CAD build for the part. Positions are in the model's coordinates, mm. A direction names the side the tool comes from. Coordinates: 2 decimals unless noted, no trailing zeros. Loops run counter-clockwise (first coordinate to the right, second up) from the corner with the lowest first, then second, coordinate; pieces in that order, holes last. Notation, with made-up numbers: (65, 70.5) -> (102, 70.5) arc R14 cw to (102, 86.5) -> close; hole circle Ø4 at (-5.5, 79). An arc over 180 degrees is marked (long way). Write each question's results on one line, items separated by ' | '.
from build123d import *

# Parameters (mm, degrees)
SKETCH_1_R      = 1.4
EXTRUDE_1_DEPTH = 33


with BuildPart() as part:
    # 草图1 → 凸台-拉伸1 (new body)
    with BuildSketch(Plane(origin=(0, 0, 0), x_dir=(1, 0, 0), z_dir=(0, 1, 0))):
        with BuildLine():
            Line((63.539198291, -45.541591726), (63.539198291, -25.541591726))
            Line((63.539198291, -25.541591726), (83.539198291, -25.541591726))
            ThreePointArc((83.539198291, -25.541591726), (88.539198291, -20.541591726), (83.539198291, -15.541591726))
            Line((83.539198291, -15.541591726), (49.205502665, -15.541591726))
            ThreePointArc((49.205502665, -15.541591726), (45.669968759, -17.006057821), (44.205502665, -20.541591726))
            Line((44.205502665, -20.541591726), (44.205502665, -50.541591726))
            ThreePointArc((44.205502665, -50.541591726), (45.669968759, -54.077125632), (49.205502665, -55.541591726))
            Line((49.205502665, -55.541591726), (83.539198291, -55.541591726))
            ThreePointArc((83.539198291, -55.541591726), (88.539198291, -50.541591726), (83.539198291, -45.541591726))
            Line((83.539198291, -45.541591726), (63.539198291, -45.541591726))
        make_face()
        with Locations(Location((83.539198291, -20.541591726, 0), (0, 0, 270))):
            Circle(SKETCH_1_R, mode=Mode.SUBTRACT)
        with Locations(Location((83.539198291, -50.541591726, 0), (0, 0, 90))):
            Circle(SKETCH_1_R, mode=Mode.SUBTRACT)
        with Locations(Location((51.406078432, -20.541591726, 0), (0, 0, 270))):
            Circle(SKETCH_1_R, mode=Mode.SUBTRACT)
        with Locations(Location((51.406078432, -35.541591726, 0), (0, 0, 270))):
            Circle(SKETCH_1_R, mode=Mode.SUBTRACT)
        with Locations(Location((51.406078432, -50.541591726, 0), (0, 0, 90))):
            Circle(SKETCH_1_R, mode=Mode.SUBTRACT)
    extrude(amount=EXTRUDE_1_DEPTH)


solid = part.part
1) Slice it at A-A (x = 67). Write the cut outline in (y, z).
Outcome:
outline: (0, 15.54) -> (33, 15.54) -> (33, 25.54) -> (0, 25.54) -> close; (0, 45.54) -> (33, 45.54) -> (33, 55.54) -> (0, 55.54) -> close
2) Pin check, flat tips, straight feed: pin 1 (6 mm diameter, centred on y = 24.5, z = 39.5, fed in from +X); pin 2 (1.7 mm diameter, centred on x = 83.54, z = 20.54, fed in from -Y); pin 3 (12 mm diameter, centred on y = 26.5, z = 28.5, fed in from +X). Stop position of each tip, or through.
Outcome:
pin 1: stops at x = 63.54 | pin 2: passes through | pin 3: stops at x = 88.14
3) Drill centre lines: L1, parallel to Z at x = 74, y = 21.5; L2, parallel to Z at x = 83.5, y = 22; L3, parallel to X at y = 4, z = 19.5. Where is each one in solid material? Low to high. Write a range as from..to.
Outcome:
L1: z = 15.54..25.54, 45.54..55.54 | L2: z = 15.54..19.14, 21.94..25.54, 45.54..49.14, 51.94..55.54 | L3: x = 44.32..50.47, 52.34..82.6, 84.47..88.43
4) Slice it at C-C (z = 29). Write the cut outline in (x, y), then the cut area to 3 significant figures.
Outcome:
outline: (44.21, 0) -> (63.54, 0) -> (63.54, 33) -> (44.21, 33) -> close | area: 638 mm^2
5) Which spindle directions (+Z, -Z, +X, -X, +Y, -Y) get a long thin tool onto all of the face, cutting with end or side? Do faces 4 (the flat face through (66, 16, 55.542)), 5 (the flat face through (74, 16, 45.542)). Say none if no direction does.
Outcome:
face 4: +Z, +X, -X, +Y, -Y | face 5: +X, +Y, -Y
6) Slice it at D-D (x = 47). Write the cut outline in (y, z).
Outcome:
outline: (0, 16.05) -> (33, 16.05) -> (33, 55.03) -> (0, 55.03) -> close
7) Slice it at B-B (y = 18). Write the cut outline in (x, z).
Outcome:
outline: (44.21, 20.54) arc R5 ccw to (49.21, 15.54) -> (83.54, 15.54) arc R5 ccw to (83.54, 25.54) -> (63.54, 25.54) -> (63.54, 45.54) -> (83.54, 45.54) arc R5 ccw to (83.54, 55.54) -> (49.21, 55.54) arc R5 ccw to (44.21, 50.54) -> close; hole circle Ø2.8 at (51.41, 20.54); hole circle Ø2.8 at (51.41, 35.54); hole circle Ø2.8 at (51.41, 50.54); hole circle Ø2.8 at (83.54, 20.54); hole circle Ø2.8 at (83.54, 50.54)
8) Two-plate mould, pull along Z, no slides. Class faces 1 (the flat face through (67, 16, 15.542)), 2 (the cylindrical face through (52.59, 16.27, 36.29)), 3 (the flat face through (61, 33, 35)): pulls with the +Z half, pulls with the -Z half, needs draft (parallel to the pull), parting line crosses it, or undercut.
Outcome:
face 1: pulls with the -Z half | face 2: undercut | face 3: needs draft
